Model file for the job. Use its own axes, mm. A direction names the side the tool comes from. Round coordinates to 2 decimals unless told otherwise and drop trailing zeros. Write each loop counter-clockwise with the first axis right and the second up, starting at its lowest first coordinate (ties: lowest second). Pieces come first, ordered by that corner, then holes. Notation, with made-up numbers: (17, -12) - (65, -12) arc R13 ccw to (65, 12) - close; hole circle Ø10 at (25.5, 23.25). An arc over 180 degrees is marked (long way). One line per item, written item: value.
from build123d import *

# Parameters (mm, degrees)
F0_W     = 12.7
F0_H     = 12.7
F0_W_2   = 63.5
F0_H_2   = 38.1
F1_DEPTH = 50.8
F2_W     = 25.4
F2_H     = 16.551355
F3_DEPTH = 88.9


with BuildPart() as f1:
    # F0 (on Right) → F1 (new body)
    with BuildSketch(Plane.YZ):
        with Locations((38.1, 0)):
            Rectangle(F0_W, F0_H)
        Rectangle(F0_W_2, F0_H)
        with Locations((38.1, 25.4)):
            Rectangle(F0_W, F0_H_2)
        with Locations((-38.1, 0)):
            Rectangle(F0_W, F0_H)
        with Locations((-38.1, 25.4)):
            Rectangle(F0_W, F0_H_2)
    extrude(amount=F1_DEPTH)

    # F2 (on face) → F3 (cut)
    with BuildSketch(Plane(origin=(0, 44.45, 0), x_dir=(-1, 0, 0), z_dir=(0, 1, 0))):
        with Locations((-25.4, 27.325677)):
            Rectangle(F2_W, F2_H)
    extrude(amount=-F3_DEPTH, mode=Mode.SUBTRACT)


solid = f1.part
1. Band-saw the part on C-C on x = 27. Write the cut outline in (y, z), plus the area to 3 significant figures.
Report:
outline: (-44.45, -6.35) - (44.45, -6.35) - (44.45, 19.05) - (31.75, 19.05) - (31.75, 6.35) - (-31.75, 6.35) - (-31.75, 19.05) - (-44.45, 19.05) - close; (-44.45, 35.6) - (-31.75, 35.6) - (-31.75, 44.45) - (-44.45, 44.45) - close; (31.75, 35.6) - (44.45, 35.6) - (44.45, 44.45) - (31.75, 44.45) - close
area: 1,680 mm²
2. Tool access for faces 4 (the face through (25, 31.75, 17)), 5 (the face through (50.8, -1, 2)), 6 (the face through (26, 38, 19.05)): list every direction of +Z, -Z, +X, -X, +Y, -Y with a clear straight run to the whole face (end or side of a thin tool).
Report:
face 4: +Z, +X, -X
face 5: +Z, -Z, +X, +Y, -Y
face 6: +Y, -Y
3. Band-saw the part on D-D on z = 8. Write the cut outline in (x, y), plus the area to 3 significant figures.
Report:
outline: (0, -44.45) - (50.8, -44.45) - (50.8, -31.75) - (0, -31.75) - close; (0, 31.75) - (50.8, 31.75) - (50.8, 44.45) - (0, 44.45) - close
area: 1,290 mm²
4. Wall check: probe 1 along Y at (x, z) = (11, 9); probe 2 along X at (y, z) = (-36, 28); probe 3 along Z at (x, y) = (13.5, -37.5). Give the ranges that are in metal, low to high. Write a range as [from, to].
Report:
probe 1: [-44.45, -31.75], [31.75, 44.45]
probe 2: [0, 12.7], [38.1, 50.8]
probe 3: [-6.35, 19.05], [35.6, 44.45]
5. Mould opens along X. For faces 1 (the face through (38.1, 38, 27)), 2 (the face through (0, -1, 2)), 3 (the face through (25, 0, 6.35)) say: released by +X, released by -X, zero draft, split by the parting line, or undercut.
Report:
face 1: undercut
face 2: released by -X
face 3: zero draft
6. Drop flat-ended pins along their axis: pin 1 (8 mm diameter, centred on x = 32, z = 28, fed in from +Y); pin 2 (2 mm diameter, centred on x = 18.5, y = 15, fed in from +Z). Give the stop position or say it passes through.
Report:
pin 1: through
pin 2: z = 6.35
7. Band-saw the part on A-A on y = 38.5. Write the cut outline in (x, z).
Report:
outline: (0, -6.35) - (50.8, -6.35) - (50.8, 44.45) - (0, 44.45) - close; hole (12.7, 19.05) - (38.1, 19.05) - (38.1, 35.6) - (12.7, 35.6) - close
8. Band-saw the part on B-B on z = 32.5. Write the cut outline in (x, y), plus the area to 3 significant figures.
Report:
outline: (0, -44.45) - (12.7, -44.45) - (12.7, -31.75) - (0, -31.75) - close; (0, 31.75) - (12.7, 31.75) - (12.7, 44.45) - (0, 44.45) - close; (38.1, -44.45) - (50.8, -44.45) - (50.8, -31.75) - (38.1, -31.75) - close; (38.1, 31.75) - (50.8, 31.75) - (50.8, 44.45) - (38.1, 44.45) - close
area: 645 mm²
